```python
from build123d import *

# Parameters (mm, degrees)
F0_W     = 80
F0_H     = 80
F1_DEPTH = 10
F2_D     = 8.5
F4_D     = 8


with BuildPart() as f1:
    # F0 (on Front) → F1 (new body)
    with BuildSketch(Plane.XZ):
        Rectangle(F0_W, F0_H)
    extrude(amount=F1_DEPTH)

    # F2 (through all)
    with Locations(Plane(origin=(0, 0, 0), x_dir=(1, 0, 0), z_dir=(0, 1, 0))):
        with Locations((-30, 30), (30, 30), (30, -30), (-30, -30)):
            Hole(F2_D / 2)

    # F4 (through all)
    with Locations(Plane(origin=(0, 0, 0), x_dir=(1, 0, 0), z_dir=(0, 1, 0))):
        with Locations((0, 0)):
            Hole(F4_D / 2)


solid = f1.part
```
Geometry check sheet. Reference: the model listing, model coordinates, mm. Coordinates: 2 decimals unless noted, no trailing zeros. Write each loop counter-clockwise with the first axis right and the second up, starting at its lowest first coordinate (ties: lowest second). Pieces come first, ordered by that corner, then holes. Notation, with made-up numbers: (58, 52.25) -> (69, 52.25) arc R16 ccw to (69, 66.25) -> close; hole circle Ø2 at (59.25, 82.25). An arc over 180 degrees is marked (long way). Use CSV: the item, a comma, the result in double quotes. Start each with the question number.
Item 1: Cross-section at D-D, the plane z = 30. Record the cut outline in (x, y), plus the area to 3 significant figures.
Item 2: Cross-section at A-A, the plane z = 0. Record the cut outline in (x, y), plus the area to 3 significant figures.
Item 3: Cross-section at C-C, the plane y = -8.25. Record the cut outline in (x, z).
Item 4: Cross-section at B-B, the plane x = 30. Record the cut outline in (y, z), plus the area to 3 significant figures.
Item 5: Mould release check, pull along Z, two halves, no side actions. Record for faces 1 (the flat face through (-1, -5, 40)), 2 (the flat face through (-40, -5, -1)), 3 (the cylindrical face through (-26.63, -5.07, -27.41)): released by +Z, released by -Z, zero draft, split by the parting line, or undercut.
Item 6: Thickness scan on line 1 (X direction, y = -6.25, z = 30); line 2 (Z direction, x = 0, y = -4). Record the ranges inside material, lowest first.
Answers:
1,outline,"(-40, -10) -> (-34.25, -10) -> (-34.25, 0) -> (-40, 0) -> close; (-25.75, -10) -> (25.75, -10) -> (25.75, 0) -> (-25.75, 0) -> close; (34.25, -10) -> (40, -10) -> (40, 0) -> (34.25, 0) -> close"
1,area,"630 mm^2"
2,outline,"(-40, -10) -> (-4, -10) -> (-4, 0) -> (-40, 0) -> close; (4, -10) -> (40, -10) -> (40, 0) -> (4, 0) -> close"
2,area,"720 mm^2"
3,outline,"(-40, -40) -> (40, -40) -> (40, 40) -> (-40, 40) -> close; hole circle Ø8.5 at (-30, -30); hole circle Ø8.5 at (-30, 30); hole circle Ø8 at (0, 0); hole circle Ø8.5 at (30, -30); hole circle Ø8.5 at (30, 30)"
4,outline,"(-10, -40) -> (0, -40) -> (0, -34.25) -> (-10, -34.25) -> close; (-10, -25.75) -> (0, -25.75) -> (0, 25.75) -> (-10, 25.75) -> close; (-10, 34.25) -> (0, 34.25) -> (0, 40) -> (-10, 40) -> close"
4,area,"630 mm^2"
5,face 1,"released by +Z"
5,face 2,"zero draft"
5,face 3,"undercut"
6,line 1,"-40 to -34.25, -25.75 to 25.75, 34.25 to 40"
6,line 2,"-40 to -4, 4 to 40"
